Design review of the part built by this model. Coordinates are the model's own, in mm. A direction names the side the tool comes from. Give positions to 0.01 mm unless a question says otherwise; leave off trailing zeros. Order: outer loops, then holes, each group sorted by start corner. A loop starts at its lowest first (then second) coordinate and runs counter-clockwise, first axis right, second up. Notation, with made-up numbers: (86, -28) -> (124, -28) arc R25 ccw to (124, -9) -> close; hole circle Ø9 at (84.25, -34). An arc over 180 degrees is marked (long way). Use a Markdown table: item, result. Add a question column.
Autodesk Inventor part; units mm, degrees
ref_plane "YZ Plane" through (0, 0, 0) normal (1, 0, 0) x (0, 1, 0)
ref_plane "XZ Plane" through (0, 0, 0) normal (0, 1, 0) x (-1, 0, 0)
ref_plane "XY Plane" through (0, 0, 0) normal (0, 0, 1) x (1, 0, 0)
sketch "Sketch1" plane through (0, 0, 0) normal (0, 1, 0) x (-1, 0, 0)
  line L0 (-24.55, -31.25) -> (24.55, -31.25)
  line L1 (24.55, -31.25) -> (24.55, 31.25)
  line L2 (24.55, 31.25) -> (-24.55, 31.25)
  line L3 (-24.55, 31.25) -> (-24.55, -31.25)
  line L4 (-24.55, -31.25) -> (24.55, 31.25) construction
  line L5 (24.55, -31.25) -> (-24.55, 31.25) construction
  point P0 (0, 0)
  dimension "d0" = 62.5
  dimension "d1" = 49.1
extrude "Extrusion1" add sketch "Sketch1" along normal blind 6
sketch "Sketch2" plane through (0, 6, 0) normal (0, 1, 0) x (1, 0, 0)
  line L0 (22.55, 29.25) -> (-22.55, 29.25)
  line L1 (-22.55, 29.25) -> (-22.55, -29.25)
  line L2 (-22.55, -29.25) -> (22.55, -29.25)
  line L3 (22.55, -29.25) -> (22.55, 29.25)
  line L4 (22.55, 29.25) -> (-22.55, -29.25) construction
  line L5 (-22.55, 29.25) -> (22.55, -29.25) construction
  line L6 (-24.55, 31.25) -> (-24.55, -31.25)
  line L7 (-24.55, -31.25) -> (24.55, -31.25)
  point P0 (0, 0)
  dimension "d4" = 2
  dimension "d5" = 2
extrude "Extrusion2" cut sketch "Sketch2" against normal blind 1
sketch "Sketch3" plane through (0, 5, 0) normal (0, 1, 0) x (1, 0, 0)
  line L0 (22.55, 28.25) -> (-22.55, 28.25)
  line L1 (-22.55, 28.25) -> (-22.55, -28.25)
  line L2 (-22.55, -28.25) -> (22.55, -28.25)
  line L3 (22.55, -28.25) -> (22.55, 28.25)
  line L4 (22.55, 28.25) -> (-22.55, -28.25) construction
  line L5 (-22.55, 28.25) -> (22.55, -28.25) construction
  line L6 (-22.55, 29.25) -> (22.55, 29.25)
  line L7 (-22.55, -29.25) -> (-22.55, 29.25)
  point P0 (0, 0)
  dimension "d48" = 1
extrude "Extrusion3" cut sketch "Sketch3" against normal blind 3.5
sketch "Sketch9" plane through (0, 6, 0) normal (0, 1, 0) x (1, 0, 0)
  line L0 (24.55, -28.25) -> (-24.55, -28.25)
  line L1 (-24.55, -28.25) -> (-24.55, -31.25)
  line L2 (-24.55, -31.25) -> (24.55, -31.25)
  line L3 (24.55, -31.25) -> (24.55, -28.25)
  line L4 (24.55, -31.25) -> (24.55, 31.25)
  line L5 (-22.55, 29.25) -> (22.55, 29.25)
  point P0 (0, 0)
  point P1 (-21.55, 29.25)
  point P2 (21.55, 29.25)
  dimension "d36" = 57.5
extrude "Extrusion7" cut sketch "Sketch9" against normal through all
sketch "Sketch10" plane through (0, 1.5, 0) normal (0, 1, 0) x (1, 0, 0)
  line L0 (22.55, -28.25) -> (-22.55, -28.25)
  line L1 (-22.55, -28.25) -> (22.55, -28.25)
  line L2 (22.55, -28.25) -> (22.55, -27.25)
  line L3 (22.55, -27.25) -> (-22.55, -27.25)
  line L4 (-22.55, -27.25) -> (-22.55, -28.25)
  point P0 (0, 0)
  point P1 (22.55, -28.25)
  dimension "d39" = 1
extrude "Extrusion8" add sketch "Sketch10" along normal up to surface (3.5 mm away)
sketch "Sketch11" plane through (0, 1.5, 0) normal (0, 1, 0) x (1, 0, 0)
  circle A0 centre (0, 27.65) radius 1.25
  circle A1 centre (0, -26.65) radius 1.25
  line L0 (1.25, -26.65) -> (1.25, -28.25)
  line L1 (-22.55, -28.25) -> (22.55, -28.25)
  line L2 (-1.25, -26.65) -> (-1.25, -28.25)
  point P0 (0, 0)
  dimension "d42" = 2.5
  dimension "d43" = 2.5
  dimension "d44" = 54.3
  dimension "d45" = 27.65
extrude "Extrusion9" cut sketch "Sketch11" along normal through all both and the other way through all
sketch "Sketch12" plane through (0, 6, 0) normal (0, 1, 0) x (1, 0, 0)
  line L0 (24.55, 31.25) -> (-24.55, 31.25)
  line L1 (-21.55, 31.25) -> (-24.55, 28.25)
  line L2 (-24.55, 31.25) -> (-24.55, -28.25)
  point P0 (0, 0)
  dimension "d49" = 3
  dimension "d50" = 3
extrude "Extrusion10" cut sketch "Sketch12" against normal blind 10
sketch "Sketch13" plane through (-22.55, 5, 28.25) normal (0, 1, 0) x (1, 0, 0)
  line L0 (21.3, 0) -> (-2, 0)
  line L1 (0, 1) -> (21.3, 1)
  line L2 (1.5, 0) -> (5.5, 0)
  line L3 (5.5, 0) -> (5.5, 1)
  line L4 (5.5, 1) -> (1.5, 1)
  line L5 (1.5, 1) -> (1.5, 0)
  line L6 (37.1, 0) -> (41.1, 0)
  line L7 (41.1, 0) -> (41.1, 1)
  line L8 (41.1, 1) -> (37.1, 1)
  line L9 (37.1, 1) -> (37.1, 0)
  line L10 (0, 0) -> (0, 57.5)
  line L11 (45.1, 57.5) -> (45.1, 0)
  line L12 (0, 56.5) -> (21.4534, 56.5)
  line L13 (0, 57.5) -> (45.1, 57.5)
  line L14 (3.5, 56.5) -> (7.5, 56.5)
  line L15 (7.5, 56.5) -> (7.5, 57.5)
  line L16 (7.5, 57.5) -> (3.5, 57.5)
  line L17 (3.5, 57.5) -> (3.5, 56.5)
  line L18 (38.6, 56.5) -> (42.6, 56.5)
  line L19 (42.6, 56.5) -> (42.6, 57.5)
  line L20 (42.6, 57.5) -> (38.6, 57.5)
  line L21 (38.6, 57.5) -> (38.6, 56.5)
  point P0 (22.55, 28.25)
  point P1 (38.6, 57)
  point P2 (3.5, 57.5)
  point P3 (7.5, 56.5)
  point P4 (38.6, 57.5)
  point P5 (1.5, 1)
  point P6 (5.5, 0)
  dimension "d53" = 4
  dimension "d54" = 4
  dimension "d55" = 1.5
  dimension "d56" = 4
  dimension "d57" = 3.5
  dimension "d58" = 2.5
  dimension "d59" = 4
  dimension "d60" = 4
extrude "Extrusion11" cut sketch "Sketch13" against normal blind 2 contours L13 L19 L18 L21 | L0 L5 L1 L3 | L17 L13 L15 L12 | L9 L8 L7 L6
sketch "Sketch17" plane through (-24.55, 0, 28.25) normal (-1, 0, 0) x (0, 0, 1)
  line L0 (-56.5, 0) -> (0, 0)
  line L1 (-1, 1.5) -> (-56.5, 1.5)
  line L2 (-8, 0) -> (-51.5, 0)
  line L3 (-51.5, 0) -> (-51.5, 1.5)
  line L4 (-51.5, 1.5) -> (-8, 1.5)
  line L5 (-8, 1.5) -> (-8, 0)
  line L6 (0, 0) -> (0, 6)
  line L7 (-8, 1.5) -> (-6, 1.5)
  line L8 (-8, 0.5) -> (-8, 1.5)
  line L9 (-8, 0) -> (-7.25, 0.75)
  line L10 (-8, 0) -> (-6.9393, 0) construction
  line L11 (-7.25, 0.75) -> (-8, 1.5)
  line L12 (-51.5, 0) -> (-52.25, 0.75)
  line L13 (-51.5, 0) -> (-50.4393, 0) construction
  line L14 (-52.25, 0.75) -> (-51.5, 1.5)
  line L15 (-59.5, 0) -> (-59.5, 6)
  line L16 (-8, 0) -> (-51.5, 0)
  line L17 (-51.5, 1.5) -> (-8, 1.5)
  point P0 (-28.25, 0)
  dimension "d69" = 8
  dimension "d72" = 45
  dimension "d73" = 45
  dimension "d75" = 45
  dimension "d76" = 45
  dimension "d77" = 8
extrude "Extrusion13" cut sketch "Sketch17" against normal through all
extrude "Extrusion14" add sketch "Sketch17" against normal blind 4.1
equation "\"d5\" = d4"
equation "\"d43\" = d42"
equation "\"d50\" = d49"
equation "\"d73\" = d72"
equation "\"d76\" = d75"
properties part number "Module Cover" material "ABS Plastic"
1) The part is to be moulded in two halves that separate along Z. For faces 6 (the flat face through (22.55, 4, 0)), 7 (the flat face through (2, 3, -31.25)), 8 (the flat face through (1.25, 2, 28)), say which applies: +Z half, -Z half, draft (parallel to the pull), parting line (faces both ways), or undercut.
2) Add section D-D (x = 0). Give the boundary of the cut face in (y, z).
3) For L1, parallel to X at y = 3.35, z = 22; L2, parallel to Z at x = -8, y = 1.65; L3, parallel to Z at x = 7, y = 5.2, list the stretches that pass through material, from the lowest coordinate up. Write a range as [from, to].
4) Insertion check: pin 1 (4 mm diameter, centred on x = 3, z = 18, fed in from -Y); pin 2 (0.9 mm diameter, centred on x = 1, y = 4.5, fed in from +Z); pin 3 (1.2 mm diameter, centred on y = 0.5, z = -9, fed in from +X); pin 4 (10 mm diameter, centred on x = -12.5, z = 20, fed in from +Y). Each pin has a flat end and moves straight along its axis. Give the tip position at first contact, or say it passes through.
5) Machinability: for faces 1 (the flat face through (-1.25, 2, 28)), 2 (the flat face through (24, 1.5, -1)), 3 (the flat face through (-13, 2, 28.25)), 4 (the flat face through (-23, 3, -29.8)), 5 (the flat face through (-3, 1.5, 22)), which of the approach directions +Z, -Z, +X, -X, +Y, -Y give a long, thin tool a straight path to every point of the face, cutting with its end or side? Answer none if there is none.
6) Add section A-A (z = 14.5). Give the boundary of the cut face in (x, y).
7) Add section B-B (x = -14). Give the boundary of the cut face in (y, z).
8) Add section C-C (y = 3.75). Give the number of separate pieces and of enclosed holes in the cut face, then the cut area to 3 significant figures.
Worked answers:
| question | item | result |
|---|---|---|
| 1 | face 6 | undercut |
| 1 | face 7 | -Z half |
| 1 | face 8 | draft |
| 2 | outline | (0, -31.25) -> (6, -31.25) -> (6, -29.25) -> (5, -29.25) -> (5, -28.9) -> (0, -28.9) -> close; (0, -26.4) -> (1.5, -26.4) -> (1.5, -23.25) -> (0.75, -24) -> (0, -23.25) -> close; (0, 20.25) -> (0.75, 21) -> (1.5, 20.25) -> (1.5, 25.4) -> (0, 25.4) -> close |
| 3 | L1 | [-24.55, -22.55], [22.55, 24.55] |
| 3 | L2 | [-31.25, -28.25], [27.25, 28.25] |
| 3 | L3 | [-31.25, -29.25] |
| 4 | pin 1 | through |
| 4 | pin 2 | z = 28.25 |
| 4 | pin 3 | x = -20.45 |
| 4 | pin 4 | y = 1.5 |
| 5 | face 1 | +Z, +Y, -Y |
| 5 | face 2 | +X, -Y |
| 5 | face 3 | +Z, +X, -X, +Y, -Y |
| 5 | face 4 | -Z, -X, +Y, -Y |
| 5 | face 5 | +Y |
| 6 | outline | (-24.55, 0) -> (-20.45, 0) -> (-20.45, 1.5) -> (-22.55, 1.5) -> (-22.55, 6) -> (-24.55, 6) -> close; (22.55, 1.5) -> (24.55, 1.5) -> (24.55, 6) -> (22.55, 6) -> close |
| 7 | outline | (0, -31.25) -> (6, -31.25) -> (6, -29.25) -> (5, -29.25) -> (5, -28.25) -> (1.5, -28.25) -> (1.5, -23.25) -> (0.75, -24) -> (0, -23.25) -> close; (0, 20.25) -> (0.75, 21) -> (1.5, 20.25) -> (1.5, 27.25) -> (5, 27.25) -> (5, 28.25) -> (0, 28.25) -> close |
| 8 | separate pieces | 3 |
| 8 | enclosed holes | 0 |
| 8 | area | 394 mm^2 |
